from build123d import *

# Parameters (mm, degrees)
F0_W      = 812.8
F0_H      = 406.4
F1_DEPTH  = 355.6
F2_W      = 711.2
F2_H      = 304.8
F3_DEPTH  = 352.425
F4_W      = 349.25
F4_H      = 304.8
F5_DEPTH  = 47.625
F6_W      = 349.25
F6_H      = 304.8
F7_DEPTH  = 47.625
F8_W      = 349.25
F8_H      = 806.45
F9_DEPTH  = 47.625
F10_W     = 349.25
F10_H     = 806.45
F11_DEPTH = 47.625


with BuildPart() as f1:
    # F0 (on Right) → F1 (new body)
    with BuildSketch(Plane.YZ):
        Rectangle(F0_W, F0_H)
    extrude(amount=-F1_DEPTH)

    # F2 (on face) → F3 (cut)
    with BuildSketch(Plane.YZ):
        Rectangle(F2_W, F2_H)
    extrude(amount=-F3_DEPTH, mode=Mode.SUBTRACT)

    # F4 (on face) → F5 (cut)
    with BuildSketch(Plane(origin=(0, -355.6, 0), x_dir=(-1, 0, 0), z_dir=(0, 1, 0))):
        with Locations((177.8, 0)):
            Rectangle(F4_W, F4_H)
    extrude(amount=-F5_DEPTH, mode=Mode.SUBTRACT)

    # F6 (on face) → F7 (cut)
    with BuildSketch(Plane.XZ.offset(-355.6)):
        with Locations((-177.8, 0)):
            Rectangle(F6_W, F6_H)
    extrude(amount=-F7_DEPTH, mode=Mode.SUBTRACT)

    # F8 (on face) → F9 (cut)
    with BuildSketch(Plane(origin=(0, 0, 152.4), x_dir=(1, 0, 0), z_dir=(0, 0, -1))):
        with Locations((-177.8, 0)):
            Rectangle(F8_W, F8_H)
    extrude(amount=-F9_DEPTH, mode=Mode.SUBTRACT)

    # F10 (on face) → F11 (cut)
    with BuildSketch(Plane.XY.offset(-152.4)):
        with Locations((-177.8, 0)):
            Rectangle(F10_W, F10_H)
    extrude(amount=-F11_DEPTH, mode=Mode.SUBTRACT)


solid = f1.part
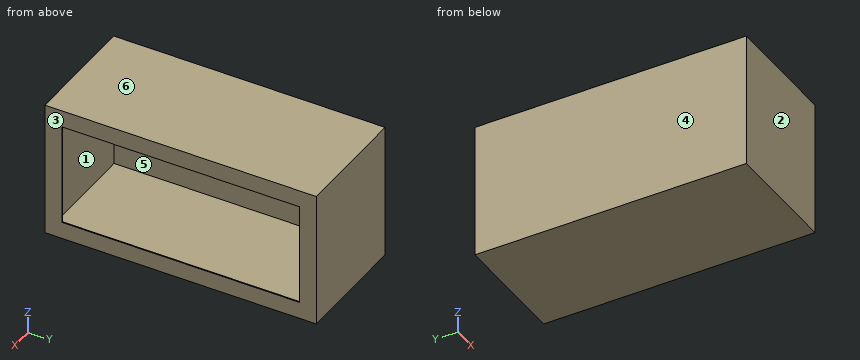
For this review, take the finished solid that the model builds, in its own axes (mm). Face numbers are marked on the shaded views. A direction names the side the tool comes from. Give positions to 0.01 mm unless a question says otherwise; leave off trailing zeros. Loops run counter-clockwise (first coordinate to the right, second up) from the corner with the lowest first, then second, coordinate; pieces in that order, holes last. Notation, with made-up numbers: M 63.25,-4 L 103.25,-4 A16 ccw 103.25,18 Z; hole C 38.5,-26 d8. An arc over 180 degrees is marked long. Answer as a JSON object with one key per item and string values. Group by question number.
Q1. Insertion check: P1, Ø1.5, axis at y = 236.5, z = -59.5, coming from the +X side (3 decimals). The pin has a flat end and moves straight along its axis. Give the tip position at first contact, or say it passes through.
Q2. Add section B-B on x = -194.5. Give the boundary of the cut face in (y, z) (3 decimals).
Q3. Add section D-D on y = 170.5. Give the boundary of the cut face in (x, z) (3 decimals), and give its area (3 significant figures).
Q4. Add section A-A on z = -162. Give the boundary of the cut face in (x, y) (3 decimals).
Q5. Add section C-C on z = 143.5. Give the boundary of the cut face in (x, y) (3 decimals).
Q6. Mouldability with a two-part tool opening along X and no side actions: class the marked faces 3, 4, 5 and 6 as +X half, -X half, draft (parallel to the pull), parting line (faces both ways), or undercut.
Q7. For probe 1 along X at (y, z) = (-181.5, -180) (3 decimals); probe 2 along Y at (x, z) = (-65, 142) (3 decimals); probe 3 along Z at (x, y) = (-72, 353) (3 decimals), list the stretches that pass through material, from the lowest coordinate up. Write a range as [from, to].
Q8. Tool access review of the marked faces 1 and 2: name each direction out of +Z, -Z, +X, -X, +Y, -Y from which nothing blocks a thin tool from reaching the whole face with its end or side.
Checked values:
{
 "1": {"P1": "x = -352.425"},
 "2": {"outline": "M -406.4,-203.2 L 406.4,-203.2 L 406.4,203.2 L -406.4,203.2 Z; hole M -403.225,-200.025 L 403.225,-200.025 L 403.225,200.025 L -403.225,200.025 Z"},
 "3": {"outline": "M -355.6,-203.2 L 0,-203.2 L 0,-152.4 L -3.175,-152.4 L -3.175,-200.025 L -352.425,-200.025 L -352.425,200.025 L -3.175,200.025 L -3.175,152.4 L 0,152.4 L 0,203.2 L -355.6,203.2 Z", "area": "3,830 mm²"},
 "4": {"outline": "M -355.6,-406.4 L 0,-406.4 L 0,406.4 L -355.6,406.4 Z; hole M -352.425,-403.225 L -3.175,-403.225 L -3.175,403.225 L -352.425,403.225 Z"},
 "5": {"outline": "M -355.6,-406.4 L 0,-406.4 L 0,-355.6 L -3.175,-355.6 L -3.175,-403.225 L -352.425,-403.225 L -352.425,403.225 L -3.175,403.225 L -3.175,355.6 L 0,355.6 L 0,406.4 L -355.6,406.4 Z"},
 "6": {"face 3": "+X half", "face 4": "-X half", "face 5": "undercut", "face 6": "draft"},
 "7": {"probe 1": "[-355.6, -352.425], [-3.175, 0]", "probe 2": "[-406.4, -403.225], [403.225, 406.4]", "probe 3": "[-203.2, -200.025], [200.025, 203.2]"},
 "8": {"face 1": "none", "face 2": "+Z, -Z, +X, -X, -Y"}
}
